```python
from build123d import *

# Parameters (mm, degrees)
SKETCH_W        = 52
SKETCH_H        = 30
PAD_DEPTH       = 6
SKETCH001_R     = 6.15
POCKET_DEPTH    = 6
SKETCH002_W     = 30
SKETCH002_H     = 2.3
POCKET001_DEPTH = 2
SKETCH003_W     = 52
SKETCH003_H     = 2.3
POCKET002_DEPTH = 2
SKETCH004_W     = 30
SKETCH004_H     = 2.3
POCKET003_DEPTH = 2
SKETCH005_W     = 52
SKETCH005_H     = 6
PAD001_DEPTH    = 20
SKETCH006_W     = 19.5
SKETCH006_H     = 3.75
POCKET004_DEPTH = 26
CHAMFER_SIZE    = 4
SKETCH007_W     = 45
SKETCH007_H     = 2
PAD002_DEPTH    = 6


with BuildPart() as part:
    # Sketch → Pad (new body)
    with BuildSketch(Plane.XY):
        Rectangle(SKETCH_W, SKETCH_H)
    extrude(amount=PAD_DEPTH)

    # Sketch001 (on Face6 of Pad) → Pocket (cut)
    with BuildSketch(Plane.XY.offset(6)):
        with Locations((-16, 6)):
            Circle(SKETCH001_R)
        with Locations((0, 6)):
            Circle(SKETCH001_R)
        with Locations((16, 6)):
            Circle(SKETCH001_R)
    extrude(amount=-POCKET_DEPTH, mode=Mode.SUBTRACT)

    # Sketch002 (on Face3 of Pocket) → Pocket001 (cut)
    with BuildSketch(Plane.YZ.offset(26)):
        with Locations((0, 3)):
            Rectangle(SKETCH002_W, SKETCH002_H)
    extrude(amount=-POCKET001_DEPTH, mode=Mode.SUBTRACT)

    # Sketch003 (on Face1 of Pocket001) → Pocket002 (cut)
    with BuildSketch(Plane(origin=(0, 15, 0), x_dir=(-1, 0, 0), z_dir=(0, 1, 0))):
        with Locations((0, 3)):
            Rectangle(SKETCH003_W, SKETCH003_H)
    extrude(amount=-POCKET002_DEPTH, mode=Mode.SUBTRACT)

    # Sketch004 (on Face6 of Pocket002) → Pocket003 (cut)
    with BuildSketch(Plane(origin=(-26, 0, 0), x_dir=(0, -1, 0), z_dir=(-1, 0, 0))):
        with Locations((0, 3)):
            Rectangle(SKETCH004_W, SKETCH004_H)
    extrude(amount=-POCKET003_DEPTH, mode=Mode.SUBTRACT)

    # Sketch005 (on Face2 of Pocket003) → Pad001 (join)
    with BuildSketch(Plane(origin=(0, 0, 0), x_dir=(1, 0, 0), z_dir=(0, 0, -1))):
        with Locations((0, 12)):
            Rectangle(SKETCH005_W, SKETCH005_H)
    extrude(amount=PAD001_DEPTH)

    # Sketch006 (on Face19 of Pad001) → Pocket004 (cut)
    with BuildSketch(Plane.XY.offset(6)):
        with Locations((1.25, -13.125)):
            Rectangle(SKETCH006_W, SKETCH006_H)
    extrude(amount=-POCKET004_DEPTH, mode=Mode.SUBTRACT)

    # Chamfer
    chamfer_edges = [part.edges().sort_by_distance(p)[0] for p in [
        (0, -9, 0),
    ]]
    chamfer(chamfer_edges, length=CHAMFER_SIZE)

    # Sketch007 (on Face19 of Chamfer) → Pad002 (join)
    with BuildSketch(Plane.XY.offset(6)):
        with Locations((0, -0.4)):
            Rectangle(SKETCH007_W, SKETCH007_H)
    extrude(amount=-PAD002_DEPTH)


solid = part.part
```
The listing builds one solid part. Answer for the finished solid, in the listing's coordinates (mm). A direction names the side the tool comes from. Coordinates: 2 decimals unless noted, no trailing zeros. Write each loop counter-clockwise with the first axis right and the second up, starting at its lowest first coordinate (ties: lowest second). Pieces come first, ordered by that corner, then holes. Notation, with made-up numbers: M 75.25,-37.75 L 91.25,-37.75 A22 ccw 91.25,-21.75 Z; hole C -36,-7.5 d10. An arc over 180 degrees is marked long. Use a Markdown table: item, result. Add a question column.
1. Section D-D (x = 0) is taken. Give the vertices of the cut face in (y, z).
2. Section B-B (x = 16) is taken. Give the vertices of the cut face in (y, z).
3. For a pull along Z with two mould halves and no side action, classify faces 4 (the flat face through (26, -10, -7)), 5 (the flat face through (24, -1, 3)), 6 (the flat face through (0, -7, -2)) as +Z half, -Z half, draft (parallel to the pull), parting line (faces both ways), or undercut.
4. Straight lines are drawn through the part: line 1 along X through (y, z) = (6, 3.65); line 2 along X through (y, z) = (6, 4.7); line 3 along Y through (x, z) = (16, 2.85). For each, find the intervals that lie inside material, in ascending order. Write a range as [from, to].
5. Section C-C (z = -12) is taken. Give the vertices of the cut face in (x, y).
6. Which of the six approach directions +Z, -Z, +X, -X, +Y, -Y give full straight-line access (tool end or side, diameter ignored) to faces 1 (the flat face through (11, -13, -7)), 2 (the flat face through (-16, 0.6, 3)), 3 (the flat face through (-24, -1, 3))?
7. Section A-A (y = 6) is taken. Give the vertices of the cut face in (x, z), plus the area to 3 significant figures.
8. Given P1, Ø12, axis at x = 4.5, z = -10.5, coming from the -Y side; P2, Ø14, axis at x = -16, y = 6, coming from the -Z side; P3, Ø8, axis at x = -7, z = -14, coming from the +Y side, each flat-ended and moving along its own axis, determine where each tip first touches the part or whether it passes through.
Data:
| question | item | result |
|---|---|---|
| 1 | outline | M -11.25,-20 L -9,-20 L -9,-4 L -5,0 L 0.6,0 L 0.6,6 L -11.25,6 Z; M 12.15,0 L 15,0 L 15,1.85 L 13,1.85 L 13,4.15 L 15,4.15 L 15,6 L 12.15,6 Z |
| 2 | outline | M -15,-20 L -9,-20 L -9,-4 L -5,0 L 0.6,0 L 0.6,6 L -15,6 Z; M 12.15,0 L 15,0 L 15,1.85 L 13,1.85 L 13,4.15 L 15,4.15 L 15,6 L 12.15,6 Z |
| 3 | face 4 | draft |
| 3 | face 5 | undercut |
| 3 | face 6 | -Z half |
| 4 | line 1 | x = [-24, -22.15], [-9.85, -6.15], [6.15, 9.85], [22.15, 24] |
| 4 | line 2 | x = [-26, -22.15], [-9.85, -6.15], [6.15, 9.85], [22.15, 26] |
| 4 | line 3 | y = [-15, 0.6], [12.15, 13] |
| 5 | outline | M -26,-15 L -8.5,-15 L -8.5,-11.25 L 11,-11.25 L 11,-15 L 26,-15 L 26,-9 L -26,-9 Z |
| 6 | face 1 | +Z, -Z, -Y |
| 6 | face 2 | +Z, -Z |
| 6 | face 3 | -X, +Y, -Y |
| 7 | outline | M -26,0 L -22.15,0 L -22.15,6 L -26,6 L -26,4.15 L -24,4.15 L -24,1.85 L -26,1.85 Z; M -9.85,0 L -6.15,0 L -6.15,6 L -9.85,6 Z; M 6.15,0 L 9.85,0 L 9.85,6 L 6.15,6 Z; M 22.15,0 L 26,0 L 26,1.85 L 24,1.85 L 24,4.15 L 26,4.15 L 26,6 L 22.15,6 Z |
| 7 | area | 81.4 mm2 |
| 8 | P1 | stops at y = -11.25 |
| 8 | P2 | stops at z = 0 |
| 8 | P3 | stops at y = -9 |
